Can you work these out from the model? Positions are in its coordinate system, mm. Face numbers are marked on the shaded views. A direction names the side the tool comes from. Give positions to 0.01 mm unless a question says otherwise; leave off trailing zeros. Write each loop counter-clockwise with the first axis right and the second up, starting at its lowest first coordinate (ties: lowest second). Pieces come first, ordered by that corner, then holes.
1. I'm going to push flat-ended pins straight in: pin 1 (10 mm diameter, centred on x = 29, z = -18.5, fed in from +Y); pin 2 (5 mm diameter, centred on x = 10, z = 0, fed in from -Y); pin 3 (1 mm diameter, centred on x = 6.5, z = 20, fed in from -Y). Where does each tip first touch, or does it pass through?
2. Suppose I cut it at A-A (y = 39). Please give me the cut outline in (x, z).
3. On a 3-axis mill with a long thin cutter (end or side, diameter ignored), from which of +Z, -Z, +X, -X, +Y, -Y can I reach the whole of each face in a straight line? I mean the marked faces 1, 2 and 3. Say none if no direction works.
4. Suppose I cut it at B-B (x = -25.5). Please give me the cut outline in (y, z), and give its area (3 significant figures).
5. Suppose I cut it at C-C (x = 25). Please give me the cut outline in (y, z).
6. If I drill on probe 1 along Z at (x, y) = (-5, 428); probe 2 along Z at (x, y) = (-0.5, 162); probe 3 along Y at (x, z) = (13.5, -16), over which ranges is the centre line in solid material (lowest first)?
Autodesk Inventor part; units mm, degrees
ref_plane "YZ Plane" through (0, 0, 0) normal (1, 0, 0) x (0, 1, 0)
ref_plane "XZ Plane" through (0, 0, 0) normal (0, 1, 0) x (-1, 0, 0)
ref_plane "XY Plane" through (0, 0, 0) normal (0, 0, 1) x (1, 0, 0)
sketch "Skizze1" plane through (0, 0, 0) normal (0, 1, 0) x (-1, 0, 0)
  circle A0 centre (0, 0) radius 40
  dimension "d0" = 80
extrude "Extrusion1" add sketch "Skizze1" along normal blind 200
sketch "Skizze2" plane through (0, 0, 0) normal (0, -1, 0) x (1, 0, 0)
  circle A0 centre (0, 0) radius 15
  dimension "d3" = 30
extrude "Extrusion2" add sketch "Skizze2" along normal blind 30
sketch "Skizze3" plane through (0, -30, 0) normal (0, -1, 0) x (1, 0, 0)
  line L0 (0, 0) -> (-7.5, 12.9904)
  circle A0 centre (0, 0) radius 15
  line L1 (0, 0) -> (-7.5, -12.9904)
  line L2 (0, 0) -> (15, 0)
  circle A1 centre (0, 0) radius 10
  point P0 (-5, -8.6603)
  point P1 (-5, 8.6603)
  point P2 (10, 0)
  dimension "d6" = 120
  dimension "d7" = 120
  dimension "d8" = 20
hole "Bohrung1" at (-5, -30, -8.6603) at (-5, -30, 8.6603) at (10, -30, 0) direction (0, 1, 0) diameter 8 depth 2 tip angle 118
mirror "Spiegeln1" about plane through (0, 200, 0) normal (0, 1, 0) of "Extrusion1", "Extrusion2", "Bohrung1"
properties part number "Foerderbandrollen"
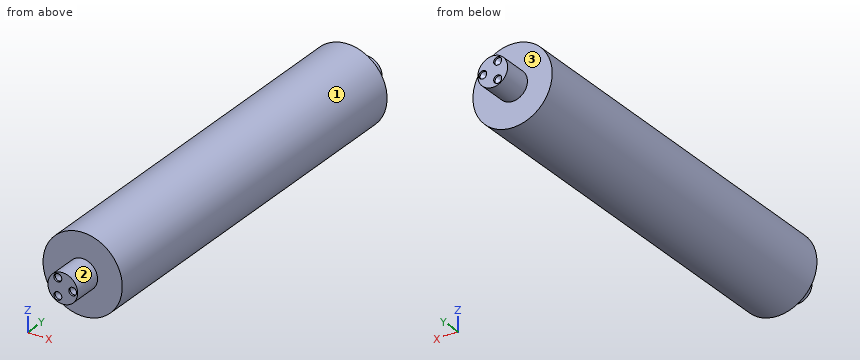
Checks:
1. pin 1: stops at y = 400
1. pin 2: stops at y = -27.1
1. pin 3: stops at y = 0
2. outline: circle Ø80 at (0, 0)
3. face 1: +Y, -Y
3. face 2: -Y
3. face 3: +Y
4. outline: (0, -30.82) - (400, -30.82) - (400, 30.82) - (0, 30.82) - close
4. area: 24,700 mm2
5. outline: (0, -31.22) - (400, -31.22) - (400, 31.22) - (0, 31.22) - close
6. probe 1: z = -14.14 to -12.66, -4.66 to 4.66, 12.66 to 14.14
6. probe 2: z = -40 to 40
6. probe 3: y = 0 to 400
